```python
from build123d import *

# Parameters (mm, degrees)
BOSS_EXTRUDE1_DEPTH = 15
SKETCH1_3_W         = 10
SKETCH1_3_H         = 15.625
BOSS_EXTRUDE2_DEPTH = 27
SKETCH2_R           = 2
CUT_EXTRUDE1_DEPTH  = 54


with BuildPart() as part:
    # Sketch1 → Boss-Extrude1 (new body, symmetric)
    with BuildSketch(Plane.XY):
        Polygon((110, -7.8125), (110, 7.8125), (101.101563673, 7.8125), (99.054231105, 2.1875), (97.402035886, 2.1875), (95.354703318, 7.8125), (93.247563673, 7.8125), (91.200231105, 2.1875), (89.548035886, 2.1875), (87.500703318, 7.8125), (85.393563673, 7.8125), (83.346231105, 2.1875), (81.694035886, 2.1875), (79.646703318, 7.8125), (77.539563673, 7.8125), (75.492231105, 2.1875), (73.840035886, 2.1875), (71.792703318, 7.8125), (69.685563673, 7.8125), (67.638231105, 2.1875), (65.986035886, 2.1875), (63.938703318, 7.8125), (61.831563673, 7.8125), (59.784231105, 2.1875), (58.132035886, 2.1875), (56.084703318, 7.8125), (53.977563673, 7.8125), (51.930231105, 2.1875), (50.278035886, 2.1875), (48.230703318, 7.8125), (46.123563673, 7.8125), (44.076231105, 2.1875), (42.424035886, 2.1875), (40.376703318, 7.8125), (38.269563673, 7.8125), (36.222231105, 2.1875), (34.570035886, 2.1875), (32.522703318, 7.8125), (30.415563673, 7.8125), (28.368231105, 2.1875), (26.716035886, 2.1875), (24.668703318, 7.8125), (22.561563673, 7.8125), (20.514231105, 2.1875), (18.862035886, 2.1875), (16.814703318, 7.8125), (14.707563673, 7.8125), (12.660231105, 2.1875), (11.008035886, 2.1875), (8.960703318, 7.8125), (6.853563673, 7.8125), (4.806231105, 2.1875), (3.154035886, 2.1875), (1.106703318, 7.8125), (-1.000436327, 7.8125), (-3.047768895, 2.1875), (-4.699964114, 2.1875), (-6.747296682, 7.8125), (-8.854436327, 7.8125), (-10.901768895, 2.1875), (-12.553964114, 2.1875), (-14.601296682, 7.8125), (-16.708436327, 7.8125), (-18.755768895, 2.1875), (-20.407964114, 2.1875), (-22.455296682, 7.8125), (-24.562436327, 7.8125), (-26.609768895, 2.1875), (-28.261964114, 2.1875), (-30.309296682, 7.8125), (-32.416436327, 7.8125), (-34.463768895, 2.1875), (-36.115964114, 2.1875), (-38.163296682, 7.8125), (-40.270436327, 7.8125), (-42.317768895, 2.1875), (-43.969964114, 2.1875), (-46.017296682, 7.8125), (-48.124436327, 7.8125), (-50.171768895, 2.1875), (-51.823964114, 2.1875), (-53.871296682, 7.8125), (-55.978436327, 7.8125), (-58.025768895, 2.1875), (-59.677964114, 2.1875), (-61.725296682, 7.8125), (-63.832436327, 7.8125), (-65.879768895, 2.1875), (-67.531964114, 2.1875), (-69.579296682, 7.8125), (-71.686436327, 7.8125), (-73.733768895, 2.1875), (-75.385964114, 2.1875), (-77.433296682, 7.8125), (-79.540436327, 7.8125), (-81.587768895, 2.1875), (-83.239964114, 2.1875), (-85.287296682, 7.8125), (-87.394436327, 7.8125), (-89.441768895, 2.1875), (-91.093964114, 2.1875), (-93.141296682, 7.8125), (-95.248436327, 7.8125), (-97.295768895, 2.1875), (-98.947964114, 2.1875), (-100.995296682, 7.8125), (-103.102436327, 7.8125), (-105.149768895, 2.1875), (-106.801964114, 2.1875), (-108.849296682, 7.8125), (-110.956436327, 7.8125), (-113.003768895, 2.1875), (-114.655964114, 2.1875), (-116.703296682, 7.8125), (-118.810436327, 7.8125), (-120, 4.54420067), (-120, -7.8125), align=None)
    extrude(amount=BOSS_EXTRUDE1_DEPTH, both=True)

    # Sketch1<3> → Boss-Extrude2 (add, symmetric)
    with BuildSketch(Plane.XY):
        with Locations((115, 0)):
            Rectangle(SKETCH1_3_W, SKETCH1_3_H)
    extrude(amount=BOSS_EXTRUDE2_DEPTH, both=True)

    # Sketch2 → Cut-Extrude1 (cut)
    with BuildSketch(Plane(origin=(120, 0, 0), x_dir=(0, 0, -1), z_dir=(1, 0, 0))):
        with Locations((-21.002491739, 0.042849803)):
            Circle(SKETCH2_R)
        with Locations((21.012499646, 0.042849803)):
            Circle(SKETCH2_R)
    extrude(amount=-CUT_EXTRUDE1_DEPTH, mode=Mode.SUBTRACT)


solid = part.part
```
Read the model definition and answer for the solid it produces. Units are mm, in the model's axes. A direction names the side the tool comes from. Round coordinates to 2 decimals unless told otherwise and drop trailing zeros. Write each loop counter-clockwise with the first axis right and the second up, starting at its lowest first coordinate (ties: lowest second). Pieces come first, ordered by that corner, then holes. Notation, with made-up numbers: M 64.5,62.25 L 68.5,62.25 A17 cw 68.5,83.25 Z; hole C -14.5,-33 d10. An arc over 180 degrees is marked long. One line per item, written item: value.
Q1. Flat-ended cylindrical pins translate along their axes: pin 1 Ø1.3 at (x, z) = (4, 1) entering from +Y; pin 2 Ø5 at (x, y) = (55.5, -6) entering from -Z; pin 3 Ø3 at (y, z) = (-2.5, 19) entering from -X. Find the tip coordinate at first contact, or state that the pin passes through.
Data:
pin 1: y = 2.19
pin 2: z = -15
pin 3: x = 110
Q2. For a pull along X with two mould halves and no side action, classify faces 1 (the flat face through (76.53, 5.04, 0.21)), 2 (the cylindrical face through (115.07, 0.131, -19.014)), 3 (the flat face through (-49.134, 5.039, 0.21)) as +X half, -X half, draft (parallel to the pull), parting line (faces both ways), or undercut.
Data:
face 1: undercut
face 2: draft
face 3: undercut
Q3. Find section A-A on y = -4.5. Write down the section's boundary in (x, z).
Data:
outline: M -120,-15 L 110,-15 L 110,-27 L 120,-27 L 120,27 L 110,27 L 110,15 L -120,15 Z
Q4. Straight lines are drawn through the part: line 1 (X direction, y = 5.75, z = 24); line 2 (Z direction, x = -84.5, y = -2.5); line 3 (Y direction, x = -27.5, z = 6). For each, find the intervals that lie inside material, in ascending order. Write a range as [from, to].
Data:
line 1: [110, 120]
line 2: [-15, 15]
line 3: [-7.81, 2.19]
Q5. Which of the six approach directions +Z, -Z, +X, -X, +Y, -Y give full straight-line access (tool end or side, diameter ignored) to faces 4 (the flat face through (-2, -7.812, 0)), 5 (the flat face through (57.123, 4.961, 0.21))?
Data:
face 4: +Z, -Z, +X, -X, -Y
face 5: +Z, -Z, +Y
